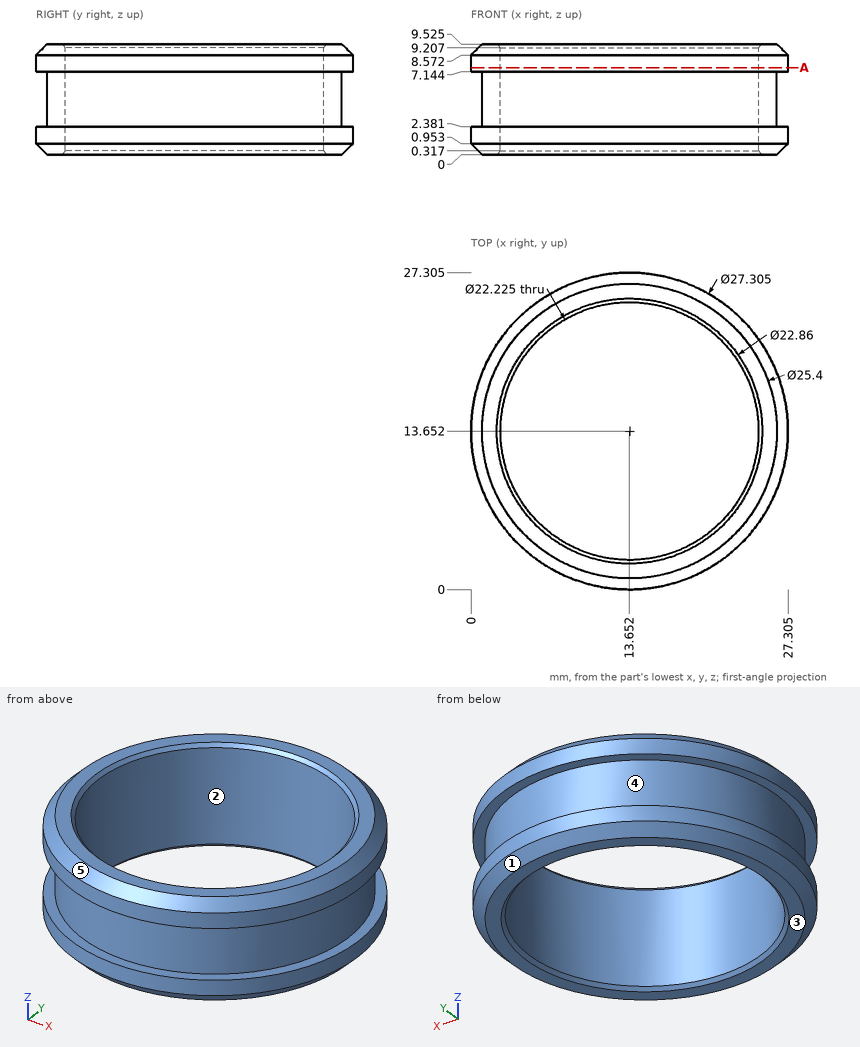
Geometry: see drawing. Coordinates: mm, zero at the bounding-box minimum. A direction names the side the tool comes from. Round coordinates to 2 decimals unless told otherwise and drop trailing zeros. Write each loop counter-clockwise with the first axis right and the second up, starting at its lowest first coordinate (ties: lowest second). Pieces come first, ordered by that corner, then holes. Notation, with made-up numbers: (26.5, 1.25) -> (41.5, 1.25) arc R16 cw to (41.5, 26.25) -> close; hole circle Ø6 at (-10.75, 47.25). An arc over 180 degrees is marked (long way). Answer as CSV lines item,"result".
1. Reachability of the marked faces 4 and 5 from +Z, -Z, +X, -X, +Y, -Y: full face, straight path, thin tool, end or side. Return the list, or none.
Geometry says:
face 4,"none"
face 5,"+Z"
2. Section A-A (z = 7.5). Return the cut outline in (x, y) (1 decimal).
Geometry says:
outline,"circle Ø27.3 at (13.7, 13.7); hole circle Ø22.2 at (13.7, 13.7)"
3. Ray query, L1, parallel to Y at x = 13.5, z = 5; L2, parallel to Y at x = 13.25, z = 8 (1 decimal); L3, parallel to X at y = 7.75, z = 3.25 (1 decimal). Return the intervals inside material, ascending. Write a range as [from, to].
Geometry says:
L1,"y = [0.95, 2.54], [24.76, 26.35]"
L2,"y = [0, 2.5], [24.8, 27.3]"
L3,"x = [2.4, 4.2], [23.1, 24.9]"
4. Mould query, pull axis Y, two halves, no side actions, for the marked faces 1, 2 and 3. Classes: +Y half, -Y half, draft (parallel to the pull), parting line (faces both ways), or undercut.
Geometry says:
face 1,"parting line"
face 2,"undercut"
face 3,"draft"
5. Contact query for flat-ended pins moving along their axis: P1, Ø5, axis at x = 24.5, y = 10, coming from the -Z side; P2, Ø5, axis at y = 5, z = 5.5, coming from the -X side (1 decimal); P3, Ø3, axis at x = 9, z = 4, coming from the -Y side; P4, Ø4, axis at y = 4.5, z = 2, coming from the +X side. Output: stop coordinate, or through.
Geometry says:
P1,"stops at z = 0"
P2,"stops at x = 1.8"
P3,"stops at y = 1.35"
P4,"stops at x = 25.28"
